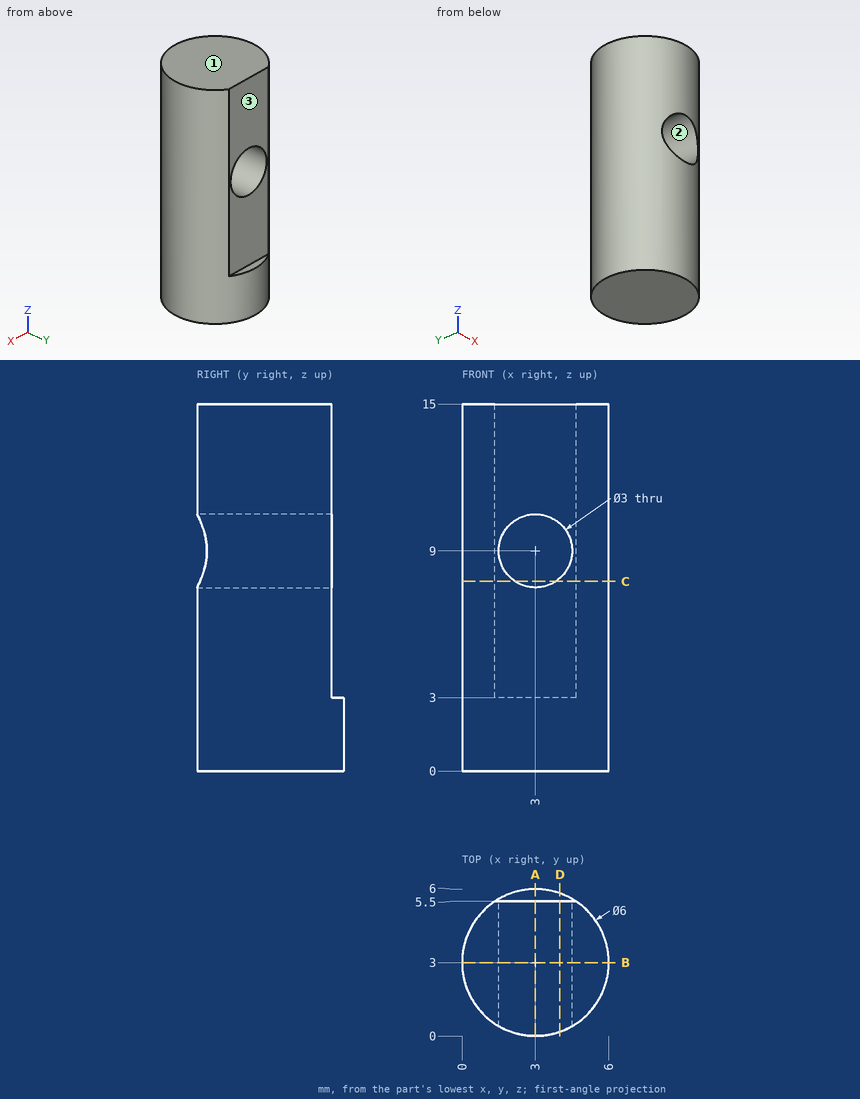
For this review, use the dimensioned drawing (mm, ordinates from the lowest corner) and the shaded views. Round coordinates to 2 decimals unless told otherwise and drop trailing zeros. Write each loop counter-clockwise with the first axis right and the second up, starting at its lowest first coordinate (ties: lowest second). Pieces come first, ordered by that corner, then holes. Notation, with made-up numbers: M 88.5,71.25 L 142.5,71.25 A17 cw 142.5,87.25 Z; hole C -17,22 d4. An arc over 180 degrees is marked long. Use CSV: the item, a comma, the result in double quotes. Start each with the question number.
(1) The part is to be moulded in two halves that separate along Z. For the marked faces 1, 2 and 3, say which applies: +Z half, -Z half, draft (parallel to the pull), parting line (faces both ways), or undercut.
(2) We need section A-A, the plane x = 3. State the section outline as (y, z) points, then the cut area to 3 significant figures.
(3) We need section B-B, the plane y = 3. State the section outline as (x, z) points.
(4) Clearance check with flat-ended pins moving along their axes: P1, Ø0.6, axis at x = 3.5, y = 6, coming from the +Z side; P2, Ø2.5, axis at x = 3, z = 9, coming from the +Y side; P3, Ø1.7, axis at x = 3, z = 11, coming from the +Y side; P4, Ø1.5, axis at y = 1.5, z = 1.5, coming from the +X side. State where each tip first meets the part, or that it passes through.
(5) We need section D-D, the plane x = 4. State the section outline as (y, z) points.
(6) We need section C-C, the plane z = 7.75. State the section outline as (x, y) points, then the cut area to 3 significant figures.
(7) For line 1 along X through (y, z) = (3.1, 9); line 2 along X through (y, z) = (4.25, 8.25); line 3 along Z through (x, y) = (3.75, 3), list the stretches that pass through material, from the lowest coordinate up.
Findings:
1,face 1,"+Z half"
1,face 2,"undercut"
1,face 3,"draft"
2,outline,"M 0,0 L 6,0 L 6,3 L 5.5,3 L 5.5,7.5 L 0,7.5 Z; M 0,10.5 L 5.5,10.5 L 5.5,15 L 0,15 Z"
2,area,"67.5 mm^2"
3,outline,"M 0,0 L 6,0 L 6,15 L 0,15 Z; hole C 3,9 d3"
4,P1,"z = 3"
4,P2,"through"
4,P3,"y = 5.5"
4,P4,"x = 5.9"
5,outline,"M 0.17,0 L 5.83,0 L 5.83,3 L 5.5,3 L 5.5,7.88 L 0.17,7.88 Z; M 0.17,10.12 L 5.5,10.12 L 5.5,15 L 0.17,15 Z"
6,outline,"M 1.34,5.5 A3 ccw 2.17,0.12 L 2.17,5.5 Z; M 3.83,0.12 A3 ccw 4.66,5.5 L 3.83,5.5 Z"
6,area,"18.1 mm^2"
7,line 1,"0 to 1.5, 4.5 to 6"
7,line 2,"0.27 to 1.7, 4.3 to 5.73"
7,line 3,"0 to 7.7, 10.3 to 15"
